from build123d import *

# Parameters (mm, degrees)
SKETCH1_R           = 2.24506403
SKETCH1_W           = 3.175
SKETCH1_H           = 3.175
BOSS_EXTRUDE1_DEPTH = 3.175


with BuildPart() as part:
    # Sketch1 → Boss-Extrude1 (new body)
    with BuildSketch(Plane(origin=(0, 0, 0), x_dir=(0, 0, -1), z_dir=(1, 0, 0))):
        with BuildLine():
            Line((-86.4616, 6.35), (0, 6.35))
            ThreePointArc((0, 6.35), (6.35, 0), (0, -6.35))
            Line((0, -6.35), (-86.4616, -6.35))
            ThreePointArc((-86.4616, -6.35), (-92.8116, 0), (-86.4616, 6.35))
        make_face()
        with Locations((-61.0616, 0)):
            Circle(SKETCH1_R, mode=Mode.SUBTRACT)
        with Locations((-86.4616, 0)):
            Circle(SKETCH1_R, mode=Mode.SUBTRACT)
        with Locations((-73.7616, 0)):
            Rectangle(SKETCH1_W, SKETCH1_H, mode=Mode.SUBTRACT)
        with BuildLine():
            Line((-54.7116, 0), (-54.7116, 1.905))
            ThreePointArc((-54.7116, 1.905), (-54.339625612, 2.803025612), (-53.4416, 3.175))
            Line((-53.4416, 3.175), (-7.62, 3.175))
            ThreePointArc((-7.62, 3.175), (-6.721974388, 2.803025612), (-6.35, 1.905))
            Line((-6.35, 1.905), (-6.35, -1.905))
            ThreePointArc((-6.35, -1.905), (-6.721974388, -2.803025612), (-7.62, -3.175))
            Line((-7.62, -3.175), (-53.4416, -3.175))
            ThreePointArc((-53.4416, -3.175), (-54.339625612, -2.803025612), (-54.7116, -1.905))
            Line((-54.7116, -1.905), (-54.7116, 0))
        make_face(mode=Mode.SUBTRACT)
        Rectangle(SKETCH1_W, SKETCH1_H, mode=Mode.SUBTRACT)
    extrude(amount=BOSS_EXTRUDE1_DEPTH)


solid = part.part
Geometry check sheet. Reference: the model listing, model coordinates, mm. A direction names the side the tool comes from. Give positions to 0.01 mm unless a question says otherwise; leave off trailing zeros. Order: outer loops, then holes, each group sorted by start corner. A loop starts at its lowest first (then second) coordinate and runs counter-clockwise, first axis right, second up. Notation, with made-up numbers: (21.25, 16) - (39.25, 16) arc R37 ccw to (39.25, 55) - close; hole circle Ø6 at (-20, -26). An arc over 180 degrees is marked (long way). Use one line per item in the form item = value.
1) Material ranges on probe 1 along Y at (x, z) = (0.6, 28.5) (3 decimals); probe 2 along Z at (x, y) = (2.15, -0.5), recorded low to high. Write a range as from..to.
Working result:
probe_1 = -6.35..-3.175, 3.175..6.35
probe_2 = -6.33..-1.59, 1.59..6.35, 54.71..58.87, 63.25..72.17, 75.35..84.27, 88.65..92.79
2) Sectioned sample at C-C (z = 10). Record the boundary of the cut face in (x, y) (3 decimals).
Working result:
outline = (0, -6.35) - (3.175, -6.35) - (3.175, -3.175) - (0, -3.175) - close; (0, 3.175) - (3.175, 3.175) - (3.175, 6.35) - (0, 6.35) - close
3) Draft check along Y on faces 3 (the face through (2, -3.175, 30)), 4 (the face through (3.175, 4, 43)), 5 (the face through (2, 6.35, 44)), 6 (the face through (1.57, -0.14, 92.81)). Enter one of: released by +Y, released by -Y, zero draft, split by the parting line, or undercut.
Working result:
face_3 = undercut
face_4 = zero draft
face_5 = released by +Y
face_6 = split by the parting line
4) Depth check by flat-ended pin: pin 1 Ø1 at (y, z) = (-3.5, 69.5) entering from -X. Enter the tip coordinate at first touch or a pass-through.
Working result:
pin_1 = 0
5) Access from +Z, -Z, +X, -X, +Y, -Y to the whole of each face (thin tool, end or side, straight path). Record for faces 1 (the face through (0, 4, 43)), 2 (the face through (2, 1.588, 0)).
Working result:
face_1 = +Z, -Z, -X, +Y, -Y
face_2 = +X, -X
6) Sectioned sample at A-A (x = 1.45). Count the separate pieces of the cut face and the enclosed holes in it, and give its area (3 significant figures).
Working result:
separate_pieces = 1
enclosed_holes = 5
area = 867 mm^2
7) Sectioned sample at D-D (y = 5). Record the boundary of the cut face in (x, z) (3 decimals).
Working result:
outline = (0, -3.914) - (3.175, -3.914) - (3.175, 90.376) - (0, 90.376) - close
